Autodesk Inventor part; units mm, degrees
ref_plane "Arbeitsebene1" through (-62.5751, -29.26, -1.7438) normal (0, 0, -1) x (0, 1, 0)
ref_plane "YZ Plane" through (0, 0, 0) normal (1, 0, 0) x (0, 1, 0)
ref_plane "XZ Plane" through (0, 0, 0) normal (0, 1, 0) x (-1, 0, 0)
sketch "Skizze1" plane through (0, 0, 0) normal (0, 0, 1) x (1, 0, 0)
  circle A0 centre (32, 0) radius 22.5
  circle A1 centre (-36, 0) radius 22.5
  line L0 (-36, -22.5) -> (32, -22.5)
  line L1 (-36, 22.5) -> (32, 22.5)
  circle A2 centre (-6, -26) radius 5.3852
  circle A3 centre (3, -27) radius 6.0828
  circle A4 centre (-1, 24) radius 2.8875
  point P0 (0, 0)
  point P1 (-10.0927, -22.5)
  point P2 (-1.9073, -22.5)
  point P3 (-1.0927, -22.5)
  point P4 (7.0927, -22.5)
  point P5 (1.4674, 22.5)
  point P6 (-3.4674, 22.5)
  dimension "d1" = 45
  dimension "d2" = 45
  dimension "d3" = 68
  dimension "d4" = 0
ref_plane "Arbeitsebene1" through (-62.5751, -29.26, -1.7438) normal (0, 0, -1) x (0, 1, 0)
extrude "Extrusion1" add sketch "Skizze1" against normal up to surface (1.7438 mm away) contours A0 | A0 L0 A3 A2 A1 L1 A4 | A1
equation "\"d2\" = d1"
Geometry check sheet. Reference: the model listing, model coordinates, mm. Give positions to 0.01 mm unless a question says otherwise; leave off trailing zeros. Write each loop counter-clockwise with the first axis right and the second up, starting at its lowest first coordinate (ties: lowest second). Pieces come first, ordered by that corner, then holes. Notation, with made-up numbers: (1.5, -19.5) - (29.5, -19.5) arc R17 ccw to (29.5, 5.5) - close; hole circle Ø2 at (85.25, 49). An arc over 180 degrees is marked (long way). Put each result on its own line as item: value.
1. Sectioned sample at C-C, the plane x = 5. Enter the section's corners in (y, z), plus the area to 3 significant figures.
Ans:
outline: (-21.26, -1.74) - (22.5, -1.74) - (22.5, 0) - (-21.26, 0) - close
area: 76.3 mm²
2. Sectioned sample at B-B, the plane y = 8. Enter the section's corners in (x, z).
Ans:
outline: (-57.03, -1.74) - (53.03, -1.74) - (53.03, 0) - (-57.03, 0) - close
3. Sectioned sample at A-A, the plane z = -0.6. Enter the section's corners in (x, y) (1 decimal).
Ans:
outline: (-36, -22.5) - (-10.1, -22.5) arc R5.4 cw to (-1.9, -22.5) - (-1.1, -22.5) arc R6.1 cw to (7.1, -22.5) - (32, -22.5) arc R22.5 ccw to (32, 22.5) - (1.5, 22.5) arc R2.9 cw to (-3.5, 22.5) - (-36, 22.5) arc R22.5 ccw to start
4. Draft check along X on faces 1 (the cylindrical face through (-58.495, 0.495, -0.86)), 2 (the cylindrical face through (54.495, -0.495, -0.86)), 3 (the cylindrical face through (-5.935, -20.615, -0.86)). Enter one of: +X half, -X half, draft (parallel to the pull), parting line (faces both ways), or undercut.
Ans:
face 1: -X half
face 2: +X half
face 3: undercut
5. Thickness scan on line 1 (X direction, y = -12, z = -0.8); line 2 (Y direction, x = 50.5, z = -0.45); line 3 (Y direction, x = -48.5, z = -1.5). Record the ranges inside material, lowest first.
Ans:
line 1: x = -55.03 to 51.03
line 2: y = -12.81 to 12.81
line 3: y = -18.71 to 18.71
6. Go/stop test with a flat-tipped pin: pin 1 (4 mm diameter, centred on x = 3, y = -6, fed in from +Z). Record where the tip stops, or that it passes through.
Ans:
pin 1: stops at z = 0
